For this review, use the dimensioned drawing (mm, ordinates from the lowest corner) and the shaded views. Coordinates: 2 decimals unless noted, no trailing zeros. Loops run counter-clockwise (first coordinate to the right, second up) from the corner with the lowest first, then second, coordinate; pieces in that order, holes last. Notation, with made-up numbers: (62, -31.75) - (88, -31.75) arc R21 ccw to (88, -25.75) - close; hole circle Ø9 at (-14, 58.25). An arc over 180 degrees is marked (long way). Use a Markdown table: item, result. Add a question column.
1) To check wall thickness, follow L1, parallel to X at y = 1.5, z = 4.25 (3 decimals); L2, parallel to Z at x = 21.5, y = 1; L3, parallel to Z at x = 93.75, y = 1.85. State the ranges of each line that lie inside material, in increasing order. Write a range as [from, to].
2) Add section A-A, the plane z = 4.25. Give the boundary of the cut face in (x, y) (3 decimals), and give its area (3 significant figures).
3) Add section D-D, the plane y = 1.85. Give the number of separate pieces and of enclosed holes in the cut face, and give its area (3 significant figures).
4) Add section B-B, the plane x = 59.5. Give the boundary of the cut face in (y, z).
5) Clearance check with a flat-ended pin moving along its axis: pin 1 (2.5 mm diameter, centred on x = 93.75, z = 19.35, fed in from -Y). State where the tip first meets the part, or that it passes through.
6) Add section C-C, the plane z = 55.1. Give the boundary of the cut face in (x, y).
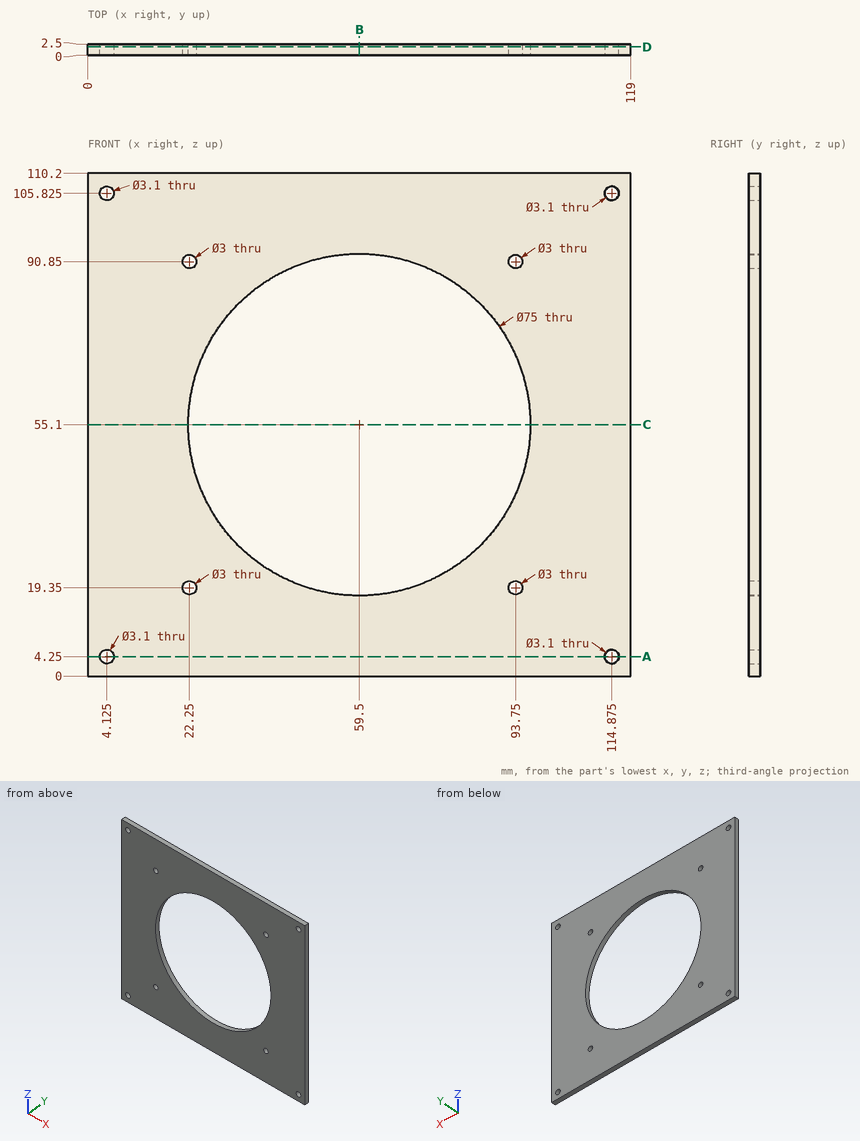
From the geometry:
| question | item | result |
|---|---|---|
| 1 | L1 | x = [0, 2.575], [5.675, 113.325], [116.425, 119] |
| 1 | L2 | z = [0, 18.05], [20.65, 89.55], [92.15, 110.2] |
| 1 | L3 | z = [0, 17.85], [20.85, 39.83], [70.37, 89.35], [92.35, 110.2] |
| 2 | outline | (0, 0) - (2.575, 0) - (2.575, 2.5) - (0, 2.5) - close; (5.675, 0) - (113.325, 0) - (113.325, 2.5) - (5.675, 2.5) - close; (116.425, 0) - (119, 0) - (119, 2.5) - (116.425, 2.5) - close |
| 2 | area | 282 mm^2 |
| 3 | separate pieces | 1 |
| 3 | enclosed holes | 9 |
| 3 | area | 8,640 mm^2 |
| 4 | outline | (0, 0) - (2.5, 0) - (2.5, 17.6) - (0, 17.6) - close; (0, 92.6) - (2.5, 92.6) - (2.5, 110.2) - (0, 110.2) - close |
| 5 | pin 1 | passes through |
| 6 | outline | (0, 0) - (22, 0) - (22, 2.5) - (0, 2.5) - close; (97, 0) - (119, 0) - (119, 2.5) - (97, 2.5) - close |
